Design review of the part shown in the three views and the two pictorial views. Dimensions are in mm from the part's minimum x, y and z. A direction names the side the tool comes from. Coordinates: 2 decimals unless noted, no trailing zeros. Write each loop counter-clockwise with the first axis right and the second up, starting at its lowest first coordinate (ties: lowest second). Pieces come first, ordered by that corner, then holes. Notation, with made-up numbers: (-8.5, 42) - (38.5, 42) arc R13 ccw to (38.5, 56) - close; hole circle Ø2 at (61, -22.75). An arc over 180 degrees is marked (long way). Write each question's results on one line, items separated by ' | '.
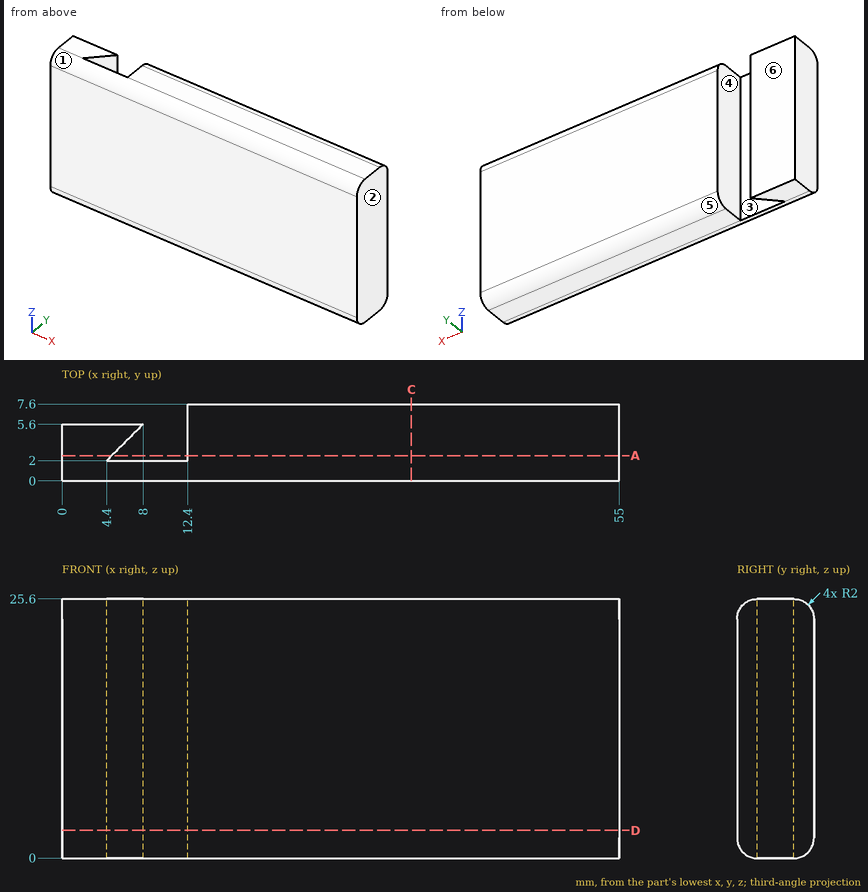
Q1. Wall thickness on line 1 along X through (y, z) = (3.5, 2.5); line 2 along X through (y, z) = (4.25, 22.75); line 3 along X through (y, z) = (5.75, 13.5): over which ranges is each line inside the solid? List them lowest first. Write a range as from..to.
Results found:
line 1: 0..5.9, 12.4..55 | line 2: 0..6.65, 12.4..55 | line 3: 12.4..55
Q2. Take a section at C-C on x = 34.5. State the section outline as (y, z) points, plus the area to 3 significant figures.
Results found:
outline: (0, 2) arc R2 ccw to (2, 0) - (5.6, 0) arc R2 ccw to (7.6, 2) - (7.6, 23.6) arc R2 ccw to (5.6, 25.6) - (2, 25.6) arc R2 ccw to (0, 23.6) - close | area: 191 mm2
Q3. Mouldability with a two-part tool opening along Y and no side actions: class the marked faces 1, 2 and 3 as pulls with the +Y half, pulls with the -Y half, needs draft (parallel to the pull), parting line crosses it, or undercut.
Results found:
face 1: pulls with the -Y half | face 2: needs draft | face 3: undercut
Q4. For pin 1 (1 mm diameter, centred on x = 24.5, z = 21.5, fed in from -Y); pin 2 (4 mm diameter, centred on x = 5, z = 7.5, fed in from +Y), all flat-tipped, find the tip position at first contact; note any pin that passes through.
Results found:
pin 1: y = 0 | pin 2: y = 5.6
Q5. For the marked faces 4, 5 and 6, list the 3-axis set-ups (+Z, -Z, +X, -X, +Y, -Y) from which the entire face can be reached by the end or side of a thin tool; tool diameter is ignored.
Results found:
face 4: +Z, -Z, +Y | face 5: -Z, +X, -X, +Y | face 6: +Z, -Z, -X, +Y
Q6. Take a section at D-D on z = 2.75. State the section outline as (x, y) points.
Results found:
outline: (0, 0) - (55, 0) - (55, 7.6) - (12.4, 7.6) - (12.4, 2) - (4.4, 2) - (8, 5.6) - (0, 5.6) - close
Q7. Take a section at A-A on y = 2.5. State the section outline as (x, z) points, plus the area to 3 significant figures.
Results found:
outline: (0, 0) - (4.9, 0) - (4.9, 25.6) - (0, 25.6) - close; (12.4, 0) - (55, 0) - (55, 25.6) - (12.4, 25.6) - close | area: 1,220 mm2
